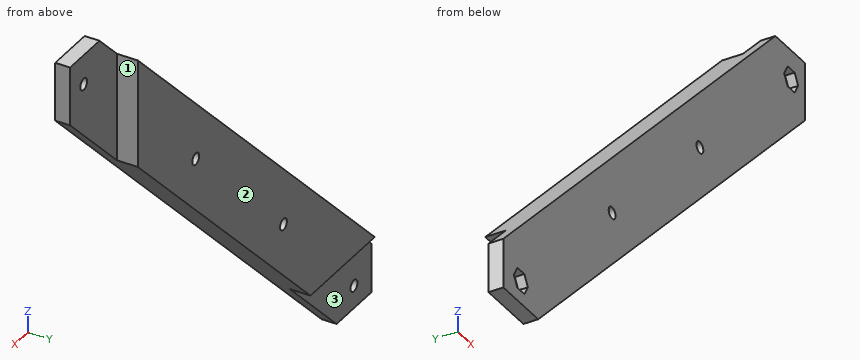
from build123d import *

# Parameters (mm, degrees)
BOSS_EXTRUDE1_DEPTH      = 12
SKETCH2_R                = 1.95
CUT_EXTRUDE1_DEPTH       = 244.540551038
SKETCH3_W                = 47
SKETCH3_H                = 27
SKETCH3_W_2              = 27
SKETCH3_H_2              = 47
CUT_EXTRUDE2_DEPTH       = 7
CUT_EXTRUDE8_DEPTH       = 244.540551038
CUT_EXTRUDE8_DEPTH_BACK  = 244.540551038
SKETCH5_R                = 1.95
CUT_EXTRUDE9_DEPTH       = 3.2
CUT_EXTRUDE10_DEPTH      = 244.540551038
CUT_EXTRUDE10_DEPTH_BACK = 244.540551038


with BuildPart() as part:
    # Sketch1 → Boss-Extrude1 (new body)
    with BuildSketch(Plane(origin=(0, 0, 0), x_dir=(1, 0, 0), z_dir=(0, 1, 0))):
        Polygon((0, 0), (20, 0), (172, -152), (172, -172), (155, -172), (0, -17), align=None)
    extrude(amount=BOSS_EXTRUDE1_DEPTH)

    # Sketch2 → Cut-Extrude1 (cut, through all)
    with BuildSketch(Plane(origin=(0, 12, 0), x_dir=(1, 0, 0), z_dir=(0, 1, 0))):
        with Locations(Location((10, -8, 0), (0, 0, 270))):
            Circle(SKETCH2_R)
        with Locations(Location((164, -162, 0), (0, 0, 270))):
            Circle(SKETCH2_R)
    extrude(amount=-CUT_EXTRUDE1_DEPTH, mode=Mode.SUBTRACT)

    # Sketch3 → Cut-Extrude2 (cut)
    with BuildSketch(Plane(origin=(0, 12, 0), x_dir=(1, 0, 0), z_dir=(0, 1, 0))):
        with Locations((23.5, -13.5)):
            Rectangle(SKETCH3_W, SKETCH3_H)
        with Locations((158.5, -148.5)):
            Rectangle(SKETCH3_W_2, SKETCH3_H_2)
    extrude(amount=-CUT_EXTRUDE2_DEPTH, mode=Mode.SUBTRACT)

    # Sketch5 → Cut-Extrude8 (cut, two sides: drawn at the far end of the back side and taken through both)
    with BuildSketch(Plane(origin=(0, 0, 0), x_dir=(1, 0, 0), z_dir=(0, 1, 0)).offset(-CUT_EXTRUDE8_DEPTH_BACK)):
        with Locations(Location((62, -60, 0), (0, 0, 270))):
            Circle(SKETCH5_R)
        with Locations(Location((112, -110, 0), (0, 0, 270))):
            Circle(SKETCH5_R)
    extrude(amount=CUT_EXTRUDE8_DEPTH + CUT_EXTRUDE8_DEPTH_BACK, mode=Mode.SUBTRACT)

    # Sketch7 → Cut-Extrude9 (cut)
    with BuildSketch(Plane.XZ):
        Polygon((13.983716857, 8), (11.991858429, 11.45), (8.008141571, 11.45), (6.016283143, 8), (8.008141571, 4.55), (11.991858429, 4.55), align=None)
        Polygon((167.983716857, 162), (165.991858429, 165.45), (162.008141571, 165.45), (160.016283143, 162), (162.008141571, 158.55), (165.991858429, 158.55), align=None)
    extrude(amount=-CUT_EXTRUDE9_DEPTH, mode=Mode.SUBTRACT)

    # Sketch8 → Cut-Extrude10 (cut, two sides: drawn at the far end of the back side and taken through both)
    with BuildSketch(Plane.XZ.offset(-CUT_EXTRUDE10_DEPTH_BACK)):
        Polygon((0, 0.25), (0, 0), (20, 0), (172, 152), (172, 172), (171.75, 172), (171.75, 152.103553391), (19.896446609, 0.25), align=None)
    extrude(amount=CUT_EXTRUDE10_DEPTH + CUT_EXTRUDE10_DEPTH_BACK, mode=Mode.SUBTRACT)


solid = part.part
Design review of the part built by this model. Coordinates are the model's own, in mm. Face numbers are marked on the shaded views. A direction names the side the tool comes from. Coordinates: 2 decimals unless noted, no trailing zeros. Order: outer loops, then holes, each group sorted by start corner. A loop starts at its lowest first (then second) coordinate and runs counter-clockwise, first axis right, second up. Notation, with made-up numbers: (-16.75, -17.5) - (3.25, -17.5) arc R13 ccw to (3.25, -7.5) - close; hole circle Ø11 at (68, 46.25). An arc over 180 degrees is marked (long way). Put each result on its own line as item: value.
1) Wall thickness on L1, parallel to X at y = 4, z = 162; L2, parallel to X at y = 5, z = 110; L3, parallel to Z at x = 62, y = 4.75: over which ranges is each line inside the solid? List them lowest first. Write a range as from..to.
Response values:
L1: x = 145..162.05, 165.95..171.75
L2: x = 93..110.05, 113.95..129.65
L3: z = 42.35..58.05, 61.95..79
2) Take a section at D-D, the plane z = 130. Give the boundary of the cut face in (x, y), and give its area (3 significant figures).
Response values:
outline: (113, 0) - (149.65, 0) - (149.65, 5) - (145, 5) - (145, 12) - (113, 12) - close
area: 407 mm²
3) Insertion check: P1, Ø13.5, axis at x = 15, z = 17, coming from the +Y side; P2, Ø5.5, axis at x = 12, z = 8, coming from the -Y side; P3, Ø3.5, axis at y = 8.5, z = 149, coming from the +X side; P4, Ø2, axis at x = 165, z = 161, coming from the -Y side. Each pin has a flat end and moves straight along its axis. Give the tip position at first contact, or say it passes through.
Response values:
P1: stops at y = 5
P2: stops at y = 0
P3: stops at x = 145
P4: stops at y = 3.2
4) Tool access review of the marked faces 1, 2 and 3: name each direction out of +Z, -Z, +X, -X, +Y, -Y from which nothing blocks a thin tool from reaching the whole face with its end or side.
Response values:
face 1: +Z, -Z, +X, +Y
face 2: +Z, -Z, +X, -X, +Y
face 3: -Z, +X, -X, +Y
5) Take a section at A-A, the plane x = 164. Give the boundary of the cut face in (y, z).
Response values:
outline: (0, 144.35) - (5, 144.35) - (5, 160.05) - (3.2, 160.05) - (3.2, 158.55) - (0, 158.55) - close; (0, 165.45) - (3.2, 165.45) - (3.2, 163.95) - (5, 163.95) - (5, 172) - (0, 172) - close
6) Take a section at B-B, the plane z = 110. Give the boundary of the cut face in (x, y).
Response values:
outline: (93, 0) - (110.05, 0) - (110.05, 12) - (93, 12) - close; (113.95, 0) - (129.65, 0) - (129.65, 12) - (113.95, 12) - close
7) Take a section at C-C, the plane x = 112. Give the boundary of the cut face in (y, z).
Response values:
outline: (0, 92.35) - (12, 92.35) - (12, 108.05) - (0, 108.05) - close; (0, 111.95) - (12, 111.95) - (12, 129) - (0, 129) - close
